Study the drawing (mm; zero at the part's minimum x, y, z) and answer. Coordinates: 2 decimals unless noted, no trailing zeros. Order: outer loops, then holes, each group sorted by start corner. A loop starts at its lowest first (then second) coordinate and runs counter-clockwise, first axis right, second up. Notation, with made-up numbers: M -8.75,13 L -0.75,13 A23 cw -0.75,37 Z; hole C 69,-21 d4. An arc over 180 degrees is marked long. Use a Markdown table: item, result. Add a question column.
1) Find section C-C on y = 2.35. Count the separate pieces of the cut face and the enclosed holes in it, plus the area to 3 significant figures.
2) This flat-tipped pin is pushed along its axis until it touches: pin 1 Ø1.9 at (x, z) = (7, 20) entering from -Y. Where does it stop, or does it pass through?
3) Find section A-A on x = 103. Write down the section's boundary in (y, z), plus the area to 3 significant figures.
4) Find the intervals of material crossed by probe 1 along Z at (x, y) = (115, 2.1); probe 2 along Z at (x, y) = (143, 1.8); probe 3 along X at (y, z) = (1.4, 37.5), in increasing order. Write a range as [from, to].
5) Find section B-B on z = 12. Write down the section's boundary in (x, y).
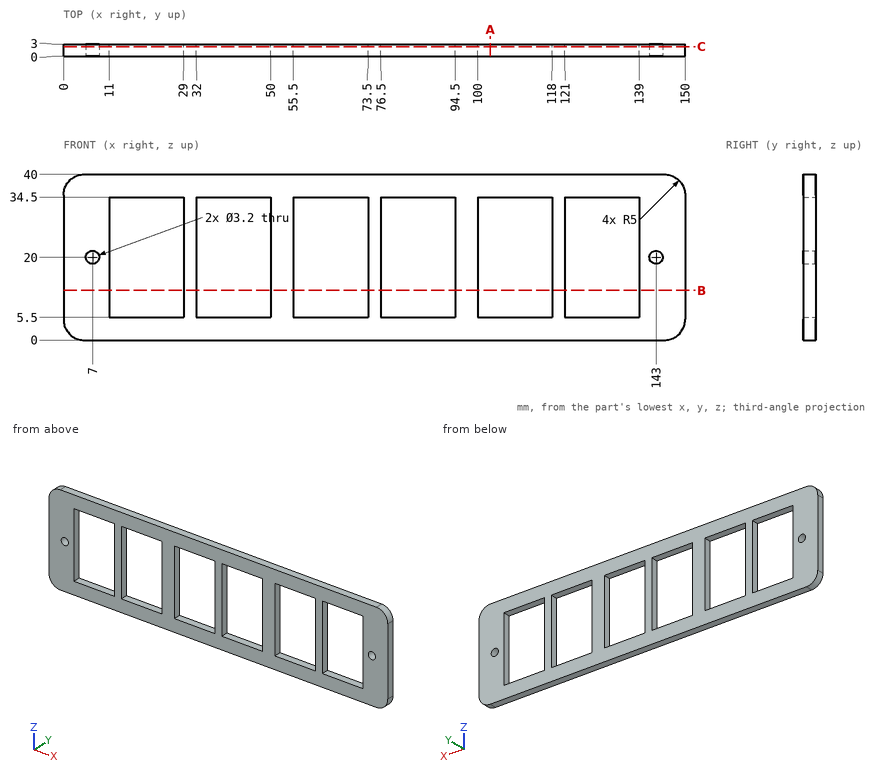
Check result:
| question | item | result |
|---|---|---|
| 1 | separate pieces | 1 |
| 1 | enclosed holes | 8 |
| 1 | area | 2,830 mm2 |
| 2 | pin 1 | passes through |
| 3 | outline | M 0,0 L 3,0 L 3,5.5 L 0,5.5 Z; M 0,34.5 L 3,34.5 L 3,40 L 0,40 Z |
| 3 | area | 33.0 mm2 |
| 4 | probe 1 | z = [0, 5.5], [34.5, 40] |
| 4 | probe 2 | z = [0, 18.4], [21.6, 40] |
| 4 | probe 3 | x = [0.67, 149.33] |
| 5 | outline | M 0,0 L 11,0 L 11,3 L 0,3 Z; M 29,0 L 32,0 L 32,3 L 29,3 Z; M 50,0 L 55.5,0 L 55.5,3 L 50,3 Z; M 73.5,0 L 76.5,0 L 76.5,3 L 73.5,3 Z; M 94.5,0 L 100,0 L 100,3 L 94.5,3 Z; M 118,0 L 121,0 L 121,3 L 118,3 Z; M 139,0 L 150,0 L 150,3 L 139,3 Z |
